Verification items for this drawing (mm, ordinates from the low corner). A direction names the side the tool comes from. Coordinates: 2 decimals unless noted, no trailing zeros. Order: outer loops, then holes, each group sorted by start corner. A loop starts at its lowest first (then second) coordinate and runs counter-clockwise, first axis right, second up.
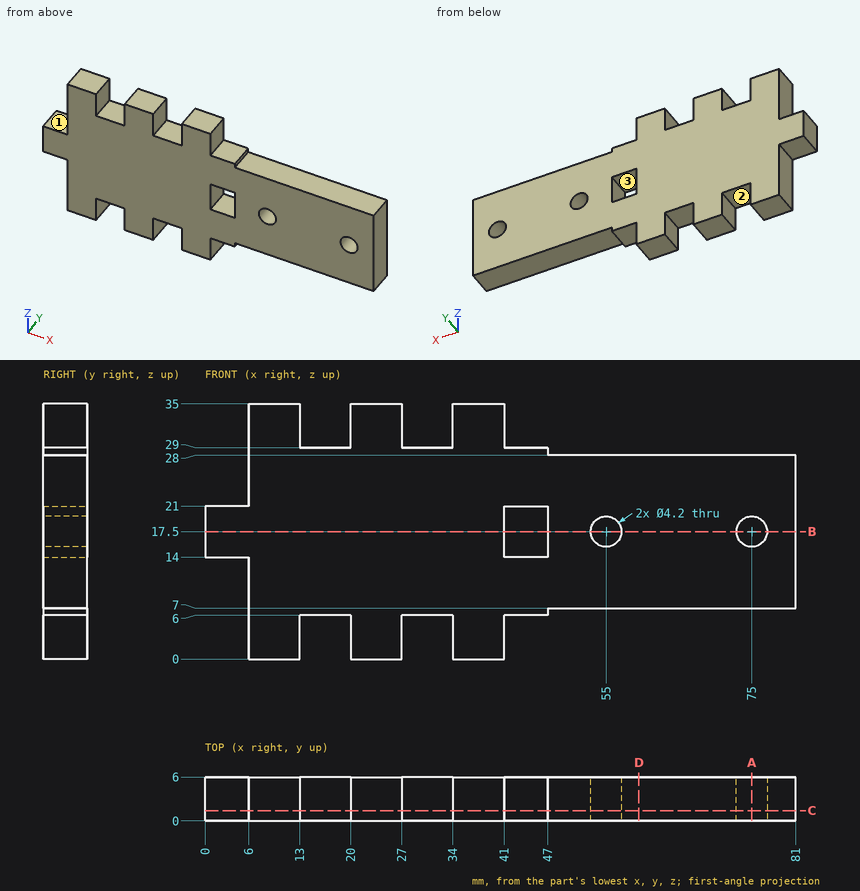
Item 1: Sectioned sample at B-B (z = 17.5). Record the cut outline in (x, y), and give its area (3 significant figures).
Item 2: Depth check by flat-ended pin: P1, Ø3, axis at y = 2, z = 2, coming from the +X side; P2, Ø1.8, axis at x = 31, y = 2.5, coming from the -Z side; P3, Ø3, axis at x = 44.5, y = 4.5, coming from the +Z side; P4, Ø3.5, axis at x = 75, z = 17.5, coming from the -Y side. Enter the tip coordinate at first touch or a pass-through.
Item 3: Sectioned sample at D-D (x = 59.5). Record the cut outline in (y, z), and give its area (3 significant figures).
Item 4: Sectioned sample at C-C (y = 1.4). Give the number of separate pieces and of enclosed holes in the cut face, and give its area (3 significant figures).
Item 5: Sectioned sample at A-A (x = 75). Record the cut outline in (y, z).
Item 6: Thickness scan on line 1 along X through (y, z) = (2.05, 5.5); line 2 along Z through (x, y) = (75, 3.25); line 3 along X through (y, z) = (3.55, 17). Record the ranges inside material, lowest first.
Item 7: Tool access check on the marked faces 1, 2 and 3. Record the directions out of +Z, -Z, +X, -X, +Y, -Y that give a thin tool (end or side, any length) a straight path to the whole face; none if there is none.
Geometry check:
1. outline: (0, 0) - (41, 0) - (41, 6) - (0, 6) - close; (47, 0) - (52.9, 0) - (52.9, 6) - (47, 6) - close; (57.1, 0) - (72.9, 0) - (72.9, 6) - (57.1, 6) - close; (77.1, 0) - (81, 0) - (81, 6) - (77.1, 6) - close
1. area: 400 mm2
2. P1: stops at x = 41
2. P2: stops at z = 6
2. P3: stops at z = 29
2. P4: passes through
3. outline: (0, 7) - (6, 7) - (6, 28) - (0, 28) - close
3. area: 126 mm2
4. separate pieces: 1
4. enclosed holes: 3
4. area: 1,880 mm2
5. outline: (0, 7) - (6, 7) - (6, 15.4) - (0, 15.4) - close; (0, 19.6) - (6, 19.6) - (6, 28) - (0, 28) - close
6. line 1: x = 6 to 13, 20 to 27, 34 to 41
6. line 2: z = 7 to 15.4, 19.6 to 28
6. line 3: x = 0 to 41, 47 to 52.96, 57.04 to 72.96, 77.04 to 81
7. face 1: +Z, -X, +Y, -Y
7. face 2: -Z, +Y, -Y
7. face 3: +Y, -Y
